from build123d import *

# Parameters (mm, degrees)
SKETCH1_R           = 5
BOSS_EXTRUDE1_DEPTH = 50
SKETCH2_R           = 2.4
BOSS_EXTRUDE2_DEPTH = 1.5
SKETCH3_R           = 2.4
BOSS_EXTRUDE3_DEPTH = 47


with BuildPart() as part:
    # Sketch1 → Boss-Extrude1 (new, symmetric)
    with BuildSketch(Plane(origin=(0, 0, 0), x_dir=(1, 0, 0), z_dir=(0, 1, 0))):
        with Locations(Location((0, 0, 0), (0, 0, 270))):
            Circle(SKETCH1_R)
    extrude(amount=BOSS_EXTRUDE1_DEPTH, both=True)

    # Sketch2 → Boss-Extrude2 (add, symmetric)
    with BuildSketch(Plane(origin=(0, 50, 0), x_dir=(1, 0, 0), z_dir=(0, 1, 0))):
        with Locations(Location((0, 0, 0), (0, 0, 270))):
            Circle(SKETCH2_R)
    boss_extrude2 = extrude(amount=BOSS_EXTRUDE2_DEPTH, both=True)

    # Mirror1: Boss-Extrude2 across plane
    add(boss_extrude2.mirror(Plane.ZX))

    # Sketch3 → Boss-Extrude3 (add)
    with BuildSketch(Plane(origin=(0, 51.5, 0), x_dir=(1, 0, 0), z_dir=(0, 1, 0))):
        with Locations(Location((0, 0, 0), (0, 0, 270))):
            Circle(SKETCH3_R)
    extrude(amount=BOSS_EXTRUDE3_DEPTH)


solid = part.part
The model under review builds one solid part; all positions refer to its coordinate system, in mm. A direction names the side the tool comes from. Give positions to 0.01 mm unless a question says otherwise; leave off trailing zeros. Write each loop counter-clockwise with the first axis right and the second up, starting at its lowest first coordinate (ties: lowest second). Pieces come first, ordered by that corner, then holes.
1. For P1, Ø1.5, axis at y = 34.5, z = 3.5, coming from the +X side; P2, Ø6, axis at y = 80, z = 0.5, coming from the +X side; P3, Ø4, axis at y = -34, z = 2.5, coming from the -X side, all flat-tipped, find the tip position at first contact; note any pin that passes through.
2. Add section B-B, the plane z = 0. Write out the cut boundary in (x, y).
3. Add section A-A, the plane x = 0. Write out the cut boundary in (y, z).
4. Wall thickness on L1, parallel to Y at x = 2.5, z = -3.5; L2, parallel to Z at x = -0.25, y = 26; L3, parallel to X at y = 57.5, z = 0.5: over which ranges is each line inside the solid? List them lowest first.
5. Add section D-D, the plane y = 86. Write out the cut boundary in (x, z), plus the area to 3 significant figures.
6. Tool access review of faces 1 (the flat face through (2.3, 50, -1.2)), 2 (the flat face through (2.3, -50, -1.2)), 3 (the cylindrical face through (-4.88, 0.7, -1.08)): name each direction out of +Z, -Z, +X, -X, +Y, -Y from which nothing blocks a thin tool from reaching the whole face with its end or side.
7. Add section C-C, the plane y = 18. Write out the cut boundary in (x, z).
Worked answers:
1. P1: stops at x = 4.18
1. P2: stops at x = 2.4
1. P3: stops at x = -4.97
2. outline: (-5, -50) - (-2.4, -50) - (-2.4, -51.5) - (2.4, -51.5) - (2.4, -50) - (5, -50) - (5, 50) - (2.4, 50) - (2.4, 98.5) - (-2.4, 98.5) - (-2.4, 50) - (-5, 50) - close
3. outline: (-51.5, -2.4) - (-50, -2.4) - (-50, -5) - (50, -5) - (50, -2.4) - (98.5, -2.4) - (98.5, 2.4) - (50, 2.4) - (50, 5) - (-50, 5) - (-50, 2.4) - (-51.5, 2.4) - close
4. L1: y = -50 to 50
4. L2: z = -4.99 to 4.99
4. L3: x = -2.35 to 2.35
5. outline: circle Ø4.8 at (0, 0)
5. area: 18.1 mm2
6. face 1: +Y
6. face 2: -Y
6. face 3: +Y, -Y
7. outline: circle Ø10 at (0, 0)
